Read the model definition and answer for the solid it produces. Units are mm, in the model's axes. Face numbers are marked on the shaded views. Coordinates: 2 decimals unless noted, no trailing zeros. Write each loop counter-clockwise with the first axis right and the second up, starting at its lowest first coordinate (ties: lowest second). Pieces come first, ordered by that corner, then holes.
(1) Section A-A on x = -11.5 is taken. Write down the section's boundary in (y, z).
(2) Given pin 1 (5.5 mm diameter, centred on x = 19, y = -11.5, fed in from +Z); pin 2 (5 mm diameter, centred on x = 19, y = 11.5, fed in from +Z); pin 3 (2 mm diameter, centred on x = -20, y = 11.5, fed in from -Z), each flat-ended and moving along its own axis, determine where each tip first touches the part or whether it passes through.
(3) Section B-B on y = 7 is taken. Write down the section's boundary in (x, z).
(4) Find the intervals of material crossed by probe 1 along Y at (x, z) = (-19, 0.75); probe 2 along Y at (x, z) = (-20.5, 1.3); probe 3 along Z at (x, y) = (3.5, -11), in increasing order.
(5) The mould has two halves that part along X. Classify the marked faces 1 and 2: +X half, -X half, draft (parallel to the pull), parting line (faces both ways), or undercut.
from build123d import *

# Parameters (mm, degrees)
F1_DEPTH     = 4
F2_R         = 1
F3_T         = -2.5
F4_T1_DEPTH  = 36
F4_T3_DEPTH  = 21
F4_T6_ANGLE  = 90
F4_T8_ANGLE  = 90
F4_T10_ANGLE = 90
F4_T12_ANGLE = 90
F5_R         = 1
F6_R         = 0.5
F7_R         = 2.15
F8_DEPTH     = 1.6


# Not quite as in the source:
# - a fillet or chamfer that OpenCascade refuses, or shapes differently, is made with other operations: its cross-section is extruded or revolved along the edge and cut away or added


with BuildPart() as f1:
    # F0 (on Top) → F1 (new body)
    with BuildSketch(Plane.XY):
        with BuildLine():
            Line((-18, -17.5), (18, -17.5))
            ThreePointArc((18, -17.5), (22.9497474683, -15.4497474683), (25, -10.5))
            Line((25, -10.5), (25, 10.5))
            ThreePointArc((25, 10.5), (22.9497474683, 15.4497474683), (18, 17.5))
            Line((18, 17.5), (-18, 17.5))
            ThreePointArc((-18, 17.5), (-22.9497474683, 15.4497474683), (-25, 10.5))
            Line((-25, 10.5), (-25, -10.5))
            ThreePointArc((-25, -10.5), (-22.9497474683, -15.4497474683), (-18, -17.5))
        make_face()
    extrude(amount=F1_DEPTH)

    # F2
    f2_edges = [f1.edges().sort_by_distance(p)[0] for p in [
        (0, -17.5, 0),
    ]]
    fillet(f2_edges, radius=F2_R)

    # F3
    f3_openings = [f1.faces().sort_by_distance(p)[0] for p in [
        (0, 0, 4),
    ]]
    offset(amount=F3_T, openings=f3_openings)

    # F4: fillet of radius 2 on 1 edges, made by hand

    # F4_s2 → F4_t1 (cut)
    with BuildSketch(Plane.YZ.offset(-18)):
        with BuildLine():
            ThreePointArc((16.9364916731, 4), (15.7117468017, 3.5811388301), (15, 2.5))
            Line((15, 2.5), (15, 4))
            Line((15, 4), (16.9364916731, 4))
        make_face()
        with BuildLine():
            ThreePointArc((-16.9364916731, 4), (-15.7117468017, 3.5811388301), (-15, 2.5))
            Line((-15, 2.5), (-15, 4))
            Line((-15, 4), (-16.9364916731, 4))
        make_face()
    extrude(amount=F4_T1_DEPTH, mode=Mode.SUBTRACT)

    # F4_s4 → F4_t3 (cut)
    with BuildSketch(Plane.XZ.offset(-10.5)):
        with BuildLine():
            ThreePointArc((-24.4364916731, 4), (-23.2117468017, 3.5811388301), (-22.5, 2.5))
            Line((-22.5, 2.5), (-22.5, 4))
            Line((-22.5, 4), (-24.4364916731, 4))
        make_face()
        with BuildLine():
            ThreePointArc((24.4364916731, 4), (23.2117468017, 3.5811388301), (22.5, 2.5))
            Line((22.5, 2.5), (22.5, 4))
            Line((22.5, 4), (24.4364916731, 4))
        make_face()
    extrude(amount=F4_T3_DEPTH, mode=Mode.SUBTRACT)

    # F4_s5 → F4_t6 (revolve, cut)
    with BuildSketch(Plane.XZ.offset(-10.5)):
        with BuildLine():
            ThreePointArc((24.4364916731, 4), (23.2117468017, 3.5811388301), (22.5, 2.5))
            Line((22.5, 2.5), (22.5, 4))
            Line((22.5, 4), (24.4364916731, 4))
        make_face()
    revolve(axis=Axis((18, 10.5, 4), (0, 0, 1)), revolution_arc=F4_T6_ANGLE, mode=Mode.SUBTRACT)

    # F4_s7 → F4_t8 (revolve, cut)
    with BuildSketch(Plane.YZ.offset(-18)):
        with BuildLine():
            ThreePointArc((16.9364916731, 4), (15.7117468017, 3.5811388301), (15, 2.5))
            Line((15, 2.5), (15, 4))
            Line((15, 4), (16.9364916731, 4))
        make_face()
    revolve(axis=Axis((-18, 10.5, 4), (0, 0, 1)), revolution_arc=F4_T8_ANGLE, mode=Mode.SUBTRACT)

    # F4_s9 → F4_t10 (revolve, cut)
    with BuildSketch(Plane.XZ.offset(10.5)):
        with BuildLine():
            ThreePointArc((-24.4364916731, 4), (-23.2117468017, 3.5811388301), (-22.5, 2.5))
            Line((-22.5, 2.5), (-22.5, 4))
            Line((-22.5, 4), (-24.4364916731, 4))
        make_face()
    revolve(axis=Axis((-18, -10.5, 4), (0, 0, 1)), revolution_arc=F4_T10_ANGLE, mode=Mode.SUBTRACT)

    # F4_s11 → F4_t12 (revolve, cut)
    with BuildSketch(Plane.YZ.offset(18)):
        with BuildLine():
            ThreePointArc((-16.9364916731, 4), (-15.7117468017, 3.5811388301), (-15, 2.5))
            Line((-15, 2.5), (-15, 4))
            Line((-15, 4), (-16.9364916731, 4))
        make_face()
    revolve(axis=Axis((18, -10.5, 4), (0, 0, 1)), revolution_arc=F4_T12_ANGLE, mode=Mode.SUBTRACT)

    # F5
    f5_edges = [f1.edges().sort_by_distance(p)[0] for p in [
        (0, 15, 2.5),
        (0, -15, 2.5),
        (21.181981, -13.681981, 2.5),
        (22.5, 0, 2.5),
        (21.181981, 13.681981, 2.5),
        (-21.181981, 13.681981, 2.5),
        (-22.5, 0, 2.5),
        (-21.181981, -13.681981, 2.5),
    ]]
    fillet(f5_edges, radius=F5_R)

    # F6
    f6_edges = [f1.edges().sort_by_distance(p)[0] for p in [
        (0, -17.5, 4),
        (-22.949747, -15.449747, 4),
        (22.949747, -15.449747, 4),
        (-25, 0, 4),
        (25, 0, 4),
        (-22.949747, 15.449747, 4),
        (22.949747, 15.449747, 4),
        (0, 17.5, 4),
    ]]
    fillet(f6_edges, radius=F6_R)

    # F7 (on face) → F8 (cut)
    with BuildSketch(Plane.XY):
        with Locations((-19, -11.5)):
            Circle(F7_R)
        with Locations((19, -11.5)):
            Circle(F7_R)
        with Locations((-19, 11.5)):
            Circle(F7_R)
        with Locations((19, 11.5)):
            Circle(F7_R)
    extrude(amount=F8_DEPTH, mode=Mode.SUBTRACT)


solid = f1.part
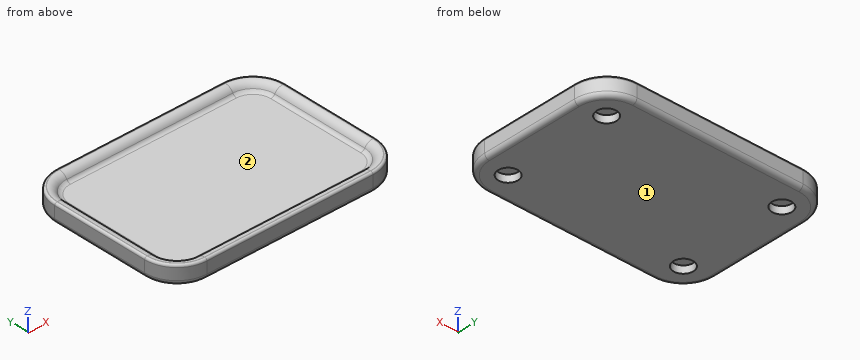
Response:
1. outline: (-17.5, 1) arc R1 ccw to (-16.5, 0) - (16.5, 0) arc R1 ccw to (17.5, 1) - (17.5, 3.5) arc R0.5 ccw to (17, 4) - (16.94, 4) arc R2 ccw to (15.2, 3) arc R1 cw to (14.34, 2.5) - (-14.34, 2.5) arc R1 cw to (-15.2, 3) arc R2 ccw to (-16.94, 4) - (-17, 4) arc R0.5 ccw to (-17.5, 3.5) - close
2. pin 1: stops at z = 2.55
2. pin 2: stops at z = 2.5
2. pin 3: stops at z = 1.6
3. outline: (-25, 1) arc R1 ccw to (-24, 0) - (24, 0) arc R1 ccw to (25, 1) - (25, 3.5) arc R0.5 ccw to (24.5, 4) - (24.44, 4) arc R2 ccw to (22.7, 3) arc R1 cw to (21.84, 2.5) - (-21.84, 2.5) arc R1 cw to (-22.7, 3) arc R2 ccw to (-24.44, 4) - (-24.5, 4) arc R0.5 ccw to (-25, 3.5) - close
4. probe 1: y = -17.4 to -13.65, -9.35 to 9.35, 13.65 to 17.4
4. probe 2: y = -17.04 to -13.04, -9.96 to 9.96, 13.04 to 17.04
4. probe 3: z = 0 to 2.5
5. face 1: draft
5. face 2: undercut
